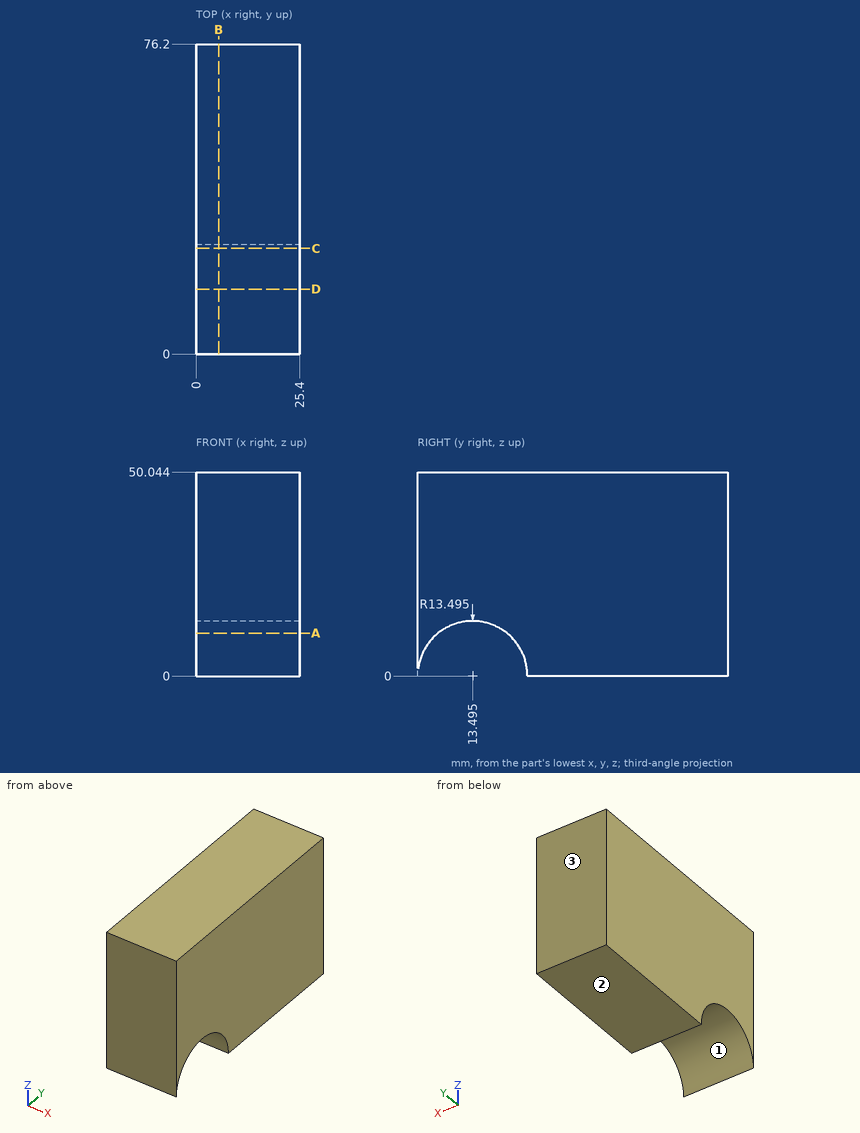
Source: three-view drawing plus pictorial views. Frame: mm from the lowest corner of the part. Coordinates: 2 decimals unless noted, no trailing zeros. Order: outer loops, then holes, each group sorted by start corner. A loop starts at its lowest first (then second) coordinate and runs counter-clockwise, first axis right, second up. Notation, with made-up numbers: M 88.25,-19.75 L 136.25,-19.75 A11 cw 136.25,-3.75 Z; hole C -24.5,4 d10. An arc over 180 degrees is marked long. One line per question, with ' | ' between items. Start each with the question number.
Item 1: Cut plane A-A, the plane z = 10.5. Return the cut outline in (x, y).
Item 2: Draft query along Y for the marked faces 1, 2 and 3. Return one class per face: released by +Y, released by -Y, zero draft, split by the parting line, or undercut.
Item 3: Cut plane B-B, the plane x = 5.5. Return the cut outline in (y, z) (1 decimal), then the cut area to 3 significant figures.
Item 4: Pin query (flat end, axial travel): pin 1 Ø10 at (x, y) = (10, 36) entering from -Z. Return the tip coordinate at first contact, or that it passes through.
Item 5: Ray query, probe 1 along Y at (x, z) = (19.25, 5); probe 2 along Y at (x, z) = (11.75, 6.5); probe 3 along Z at (x, y) = (11, 23) (1 decimal). Return the intervals inside material, ascending. Write a range as [from, to].
Item 6: Cut plane D-D, the plane y = 16. Return the cut outline in (x, z).
Item 7: Cut plane C-C, the plane y = 26. Return the cut outline in (x, z) (1 decimal).
A:
1) outline: M 0,0 L 25.4,0 L 25.4,5.02 L 0,5.02 Z; M 0,21.97 L 25.4,21.97 L 25.4,76.2 L 0,76.2 Z
2) face 1: undercut | face 2: zero draft | face 3: released by +Y
3) outline: M 0,0 A13.5 cw 27,0 L 76.2,0 L 76.2,50 L 0,50 Z | area: 3,530 mm2
4) pin 1: stops at z = 0
5) probe 1: y = [0, 0.96], [26.03, 76.2] | probe 2: y = [0, 1.67], [25.32, 76.2] | probe 3: z = [9.6, 50]
6) outline: M 0,13.26 L 25.4,13.26 L 25.4,50.04 L 0,50.04 Z
7) outline: M 0,5.1 L 25.4,5.1 L 25.4,50 L 0,50 Z
